```python
from build123d import *

# Parameters (mm, degrees)
F0_R     = 9.525
F6_DEPTH = 99.06
F7_R     = 4.1275
F1_DEPTH = 4.064
F3_R     = 4.1275
F8_DEPTH = 4.064
F4_R     = 2.9845
F9_DEPTH = 107.189
F5_SIZE  = 0.508


with BuildPart() as f6:
    # F0 (on Right) → F6 (new body)
    with BuildSketch(Plane.YZ):
        with Locations((609.6, 0)):
            Circle(F0_R)
    extrude(amount=F6_DEPTH)

    # F7 (on face) → F1 (join)
    with BuildSketch(Plane.YZ.offset(99.06)):
        with Locations((609.6, 0)):
            Circle(F7_R)
    extrude(amount=F1_DEPTH)

    # F3 (on face) → F8 (join)
    with BuildSketch(Plane(origin=(0, 0, 0), x_dir=(0, -1, 0), z_dir=(-1, 0, 0))):
        with Locations((-609.6, 0)):
            Circle(F3_R)
    extrude(amount=F8_DEPTH)

    # F4 (on face) → F9 (cut, through all)
    with BuildSketch(Plane(origin=(-4.064, 0, 0), x_dir=(0, -1, 0), z_dir=(-1, 0, 0))):
        with Locations((-609.6, 0)):
            Circle(F4_R)
    extrude(amount=-F9_DEPTH, mode=Mode.SUBTRACT)

    # F5
    f5_edges = [f6.edges().sort_by_distance(p)[0] for p in [
        (99.06, 600.075, 0),
        (0, 600.075, 0),
        (-4.064, 613.7275, 0),
        (103.124, 605.4725, 0),
    ]]
    chamfer(f5_edges, length=F5_SIZE)


solid = f6.part
```
The model under review builds one solid part; all positions refer to its coordinate system, in mm. A direction names the side the tool comes from. Round coordinates to 2 decimals unless told otherwise and drop trailing zeros. Order: outer loops, then holes, each group sorted by start corner. A loop starts at its lowest first (then second) coordinate and runs counter-clockwise, first axis right, second up.
(1) Wall thickness on L1, parallel to Z at x = 37.5, y = 609.6 (1 decimal); L2, parallel to X at y = 611.5, z = 8.25; L3, parallel to Y at x = 96, z = 0.5: over which ranges is each line inside the solid? List them lowest first.
Working result:
L1: z = -9.5 to -3, 3 to 9.5
L2: x = 0 to 99.06
L3: y = 600.09 to 606.66, 612.54 to 619.11
(2) Tool access review of faces 4 (the face through (103.124, 608, 3)), 5 (the face through (99.06, 611.5, -3.9)): name each direction out of +Z, -Z, +X, -X, +Y, -Y from which nothing blocks a thin tool from reaching the whole face with its end or side.
Working result:
face 4: +Z, -Z, +X, +Y, -Y
face 5: +X
(3) Take a section at B-B, the plane z = 0. State the section outline as (x, y) points (1 decimal).
Working result:
outline: (-4.1, 606) - (-3.6, 605.5) - (0, 605.5) - (0, 600.6) - (0.5, 600.1) - (98.6, 600.1) - (99.1, 600.6) - (99.1, 605.5) - (102.6, 605.5) - (103.1, 606) - (103.1, 606.6) - (-4.1, 606.6) - close; (-4.1, 612.6) - (103.1, 612.6) - (103.1, 613.2) - (102.6, 613.7) - (99.1, 613.7) - (99.1, 618.6) - (98.6, 619.1) - (0.5, 619.1) - (0, 618.6) - (0, 613.7) - (-3.6, 613.7) - (-4.1, 613.2) - close
(4) Mouldability with a two-part tool opening along Y and no side actions: class faces 1 (the face through (0, 611.5, -3.9)), 2 (the face through (-1.753, 613.724, 0.181)), 3 (the face through (48.78, 611.968, -1.816)) as released by +Y, released by -Y, zero draft, split by the parting line, or undercut.
Working result:
face 1: zero draft
face 2: split by the parting line
face 3: undercut
(5) For P1, Ø10, axis at y = 604, z = 7, coming from the -X side; P2, Ø5, axis at y = 615, z = 6.5, coming from the +X side; P3, Ø6, axis at x = 24, y = 616, coming from the -Z side, all flat-tipped, find the tip position at first contact; note any pin that passes through.
Working result:
P1: stops at x = -3.72
P2: stops at x = 99.06
P3: stops at z = -8.9
(6) Take a section at A-A, the plane y = 609.6. State the section outline as (x, z) points (1 decimal).
Working result:
outline: (-4.1, -3.6) - (-3.6, -4.1) - (0, -4.1) - (0, -9) - (0.5, -9.5) - (98.6, -9.5) - (99.1, -9) - (99.1, -4.1) - (102.6, -4.1) - (103.1, -3.6) - (103.1, -3) - (-4.1, -3) - close; (-4.1, 3) - (103.1, 3) - (103.1, 3.6) - (102.6, 4.1) - (99.1, 4.1) - (99.1, 9) - (98.6, 9.5) - (0.5, 9.5) - (0, 9) - (0, 4.1) - (-3.6, 4.1) - (-4.1, 3.6) - close
